```python
from build123d import *

# Parameters (mm, degrees)
BOSS_EXTRUDE1_DEPTH = 7.9248
SKETCH2_R           = 4.6355
BOSS_EXTRUDE2_DEPTH = 11.303
SKETCH6_R           = 3.9624


with BuildPart() as part:
    # Sketch1 → Boss-Extrude1 (new body, symmetric)
    with BuildSketch(Plane.XY):
        with BuildLine():
            Line((-27.441594764, 6.35), (-27.441594764, -6.35))
            Line((-27.441594764, -6.35), (-4.72195802, -14.00836494))
            ThreePointArc((-4.72195802, -14.00836494), (14.7828, 0), (-4.72195802, 14.00836494))
            Line((-4.72195802, 14.00836494), (-27.441594764, 6.35))
        make_face()
    extrude(amount=BOSS_EXTRUDE1_DEPTH, both=True)

    # Sketch2 → Boss-Extrude2 (add)
    with BuildSketch(Plane.ZY.offset(27.441594764)):
        Circle(SKETCH2_R)
    extrude(amount=BOSS_EXTRUDE2_DEPTH)

    # Sketch6 → Cut-Revolve1 (revolve, cut)
    with BuildSketch(Plane(origin=(0, 0, 0), x_dir=(0, 0, -1), z_dir=(1, 0, 0))):
        with Locations((0, 14.7828)):
            Circle(SKETCH6_R)
    revolve(axis=Axis((0, 0, 0), (0, 0, -1)), mode=Mode.SUBTRACT)


solid = part.part
```
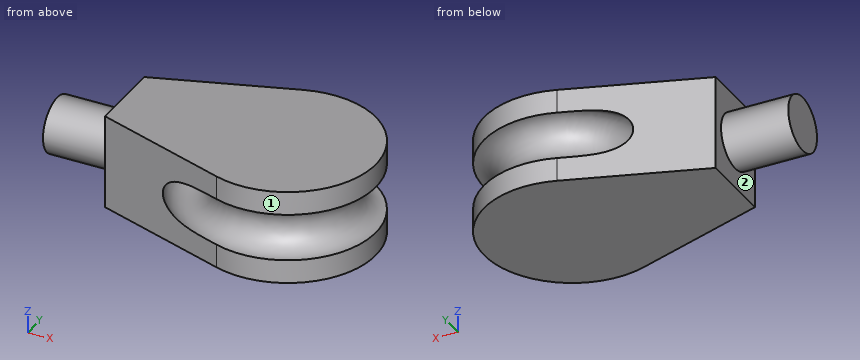
Verification items for the finished model (mm, model axes). Face numbers are marked on the shaded views. A direction names the side the tool comes from. Round coordinates to 2 decimals unless told otherwise and drop trailing zeros. Loops run counter-clockwise (first coordinate to the right, second up) from the corner with the lowest first, then second, coordinate; pieces in that order, holes last. Notation, with made-up numbers: (72, 64.25) -> (130, 64.25) arc R9 ccw to (130, 72.25) -> close; hole circle Ø6 at (36, 67.25). An arc over 180 degrees is marked (long way). Answer as a JSON object with one key per item and string values.
Q1. Section check A-A (y = 0). Record the boundary of the cut face in (x, z), then the cut area to 3 significant figures.
Data:
{"outline": "(-38.74, -4.64) -> (-27.44, -4.64) -> (-27.44, -7.92) -> (14.78, -7.92) -> (14.78, -3.96) arc R3.96 cw to (14.78, 3.96) -> (14.78, 7.92) -> (-27.44, 7.92) -> (-27.44, 4.64) -> (-38.74, 4.64) -> close; hole circle Ø7.92 at (-14.78, 0)", "area": "700 mm2"}
Q2. Access from +Z, -Z, +X, -X, +Y, -Y to the whole of each face (thin tool, end or side, straight path). Record for the marked faces 1 and 2.
Data:
{"face 1": "+Z, -Z", "face 2": "-X"}
Q3. Scan lines: line 1 (X direction, y = 1.75, z = 2.75); line 2 (X direction, y = 6, z = -1); line 3 (Y direction, x = -17, z = 0.25). Record each from-to range of solid material in increasing order. Write a range as from..to.
Data:
{"line 1": "x = -38.74..-17.55, -11.8..11.8", "line 2": "x = -27.44..-17.62, -9.16..9.16", "line 3": "y = -9.87..-7.88, 7.88..9.87"}
Q4. Section check B-B (z = 0). Record the boundary of the cut face in (x, y), then the cut area to 3 significant figures.
Data:
{"outline": "(-38.74, -4.64) -> (-27.44, -4.64) -> (-27.44, -6.35) -> (-15.64, -10.33) arc R18.75 cw to (-15.64, 10.33) -> (-27.44, 6.35) -> (-27.44, 4.64) -> (-38.74, 4.64) -> close; circle Ø21.64 at (0, 0)", "area": "626 mm2"}
Q5. Section check D-D (z = 6). Record the boundary of the cut face in (x, y), then the cut area to 3 significant figures.
Data:
{"outline": "(-27.44, -6.35) -> (-4.72, -14.01) arc R14.78 ccw (long way) to (-4.72, 14.01) -> (-27.44, 6.35) -> close", "area": "943 mm2"}
Q6. Go/stop test with a flat-tipped pin: P1, Ø4, axis at x = -32, z = -2, coming from the -Y side. Record where the tip stops, or that it passes through.
Data:
{"P1": "stops at y = -4.64"}
Q7. Section check C-C (x = 0). Record the boundary of the cut face in (y, z).
Data:
{"outline": "(-14.78, -7.92) -> (14.78, -7.92) -> (14.78, -3.96) arc R3.96 cw to (14.78, 3.96) -> (14.78, 7.92) -> (-14.78, 7.92) -> (-14.78, 3.96) arc R3.96 cw to (-14.78, -3.96) -> close"}
